Study the drawing (mm; zero at the part's minimum x, y, z) and answer. A direction names the side the tool comes from. Coordinates: 2 decimals unless noted, no trailing zeros. Order: outer loops, then holes, each group sorted by start corner. A loop starts at its lowest first (then second) coordinate and runs counter-clockwise, first axis right, second up. Notation, with made-up numbers: M 16.25,3.25 L 31.25,3.25 A21 ccw 31.25,26.25 Z; hole C -33.5,24.5 d9. An arc over 180 degrees is marked long. One line per item, written item: value. Start each with the question number.
Q1. The part is cut by section A-A on x = 22. Give the vertices of the cut face in (y, z).
Q2. Determine the mould class of the marked faces 1, 2 and 3 for opening direction Y: pulls with the +Y half, pulls with the -Y half, needs draft (parallel to the pull), parting line crosses it, or undercut.
Q3. Each of these flat-tipped pins is pushed along its axis until it touches: pin 1 Ø6 at (x, y) = (22, 6.5) entering from -Z; pin 2 Ø6 at (x, z) = (26, 10) entering from +Y. Where does it stop, or does it pass through?
Q4. Straight lines are drawn through the part: line 1 along Z through (x, y) = (5.5, 4); line 2 along Z through (x, y) = (40, 32); line 3 along Y through (x, z) = (22, 25). For each, find the intervals that lie inside material, in ascending order. Write a range as [from, to].
Q5. The part is cut by section C-C on y = 6.5. Give the vertices of the cut face in (x, z).
Q6. The part is cut by section D-D on x = 14. Give the vertices of the cut face in (y, z), then the cut area to 3 significant figures.
Q7. The part is cut by section B-B on z = 5.75. Give the vertices of the cut face in (x, y).
Q8. For the marked faces 4, 5 and 6, determine the directions among +Z, -Z, +X, -X, +Y, -Y from which every point of the face is accessible in a straight line to the end or side of a thin tool.
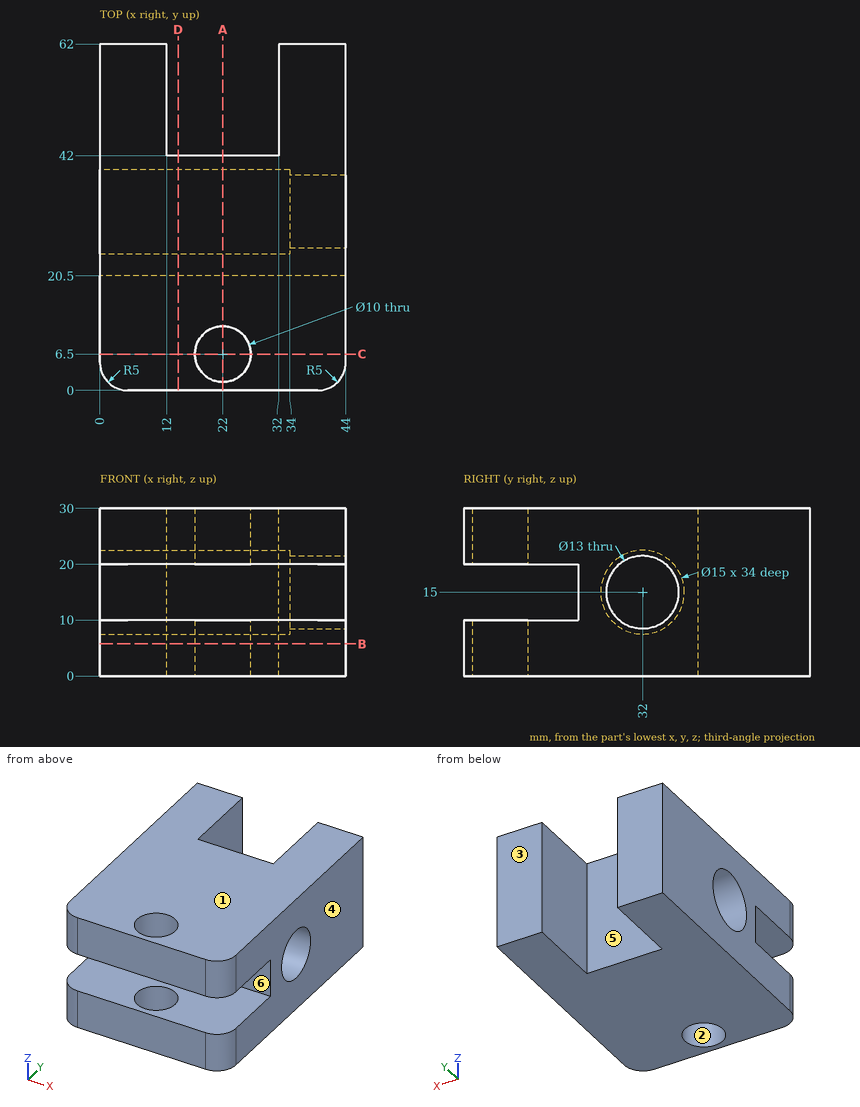
Output:
1. outline: M 0,0 L 1.5,0 L 1.5,10 L 0,10 Z; M 0,20 L 1.5,20 L 1.5,30 L 0,30 Z; M 11.5,0 L 42,0 L 42,30 L 11.5,30 L 11.5,20 L 20.5,20 L 20.5,10 L 11.5,10 Z; hole C 32,15 d15
2. face 1: needs draft
2. face 2: undercut
2. face 3: pulls with the +Y half
3. pin 1: passes through
3. pin 2: stops at y = 42
4. line 1: z = [0, 10], [20, 30]
4. line 2: z = [0, 8.5], [21.5, 30]
4. line 3: y = [0, 1.5], [11.5, 42]
5. outline: M 0,0 L 17,0 L 17,10 L 0,10 Z; M 0,20 L 17,20 L 17,30 L 0,30 Z; M 27,0 L 44,0 L 44,10 L 27,10 Z; M 27,20 L 44,20 L 44,30 L 27,30 Z
6. outline: M 0,0 L 42,0 L 42,30 L 0,30 L 0,20 L 20.5,20 L 20.5,10 L 0,10 Z; hole C 32,15 d15
6. area: 878 mm^2
7. outline: M 0,5 A5 ccw 5,0 L 39,0 A5 ccw 44,5 L 44,62 L 32,62 L 32,42 L 12,42 L 12,62 L 0,62 Z; hole C 22,6.5 d10
8. face 4: +Z, -Z, +X, +Y, -Y
8. face 5: +Z, -Z, +Y
8. face 6: +X, -X, -Y
